```python
from build123d import *

# Parameters (mm, degrees)
F0_W     = 775
F0_H     = 100
F1_DEPTH = 60
F2_W     = 775
F2_H     = 10
F3_DEPTH = 65


with BuildPart() as f1:
    # F0 (on Front) → F1 (new body)
    with BuildSketch(Plane.XZ):
        Polygon((-231.40455, 951.369763), (-301.40455, 951.369763), (-301.40455, -998.630237), (-231.40455, -998.630237), (-231.40455, -898.630237), (-231.40455, -73.630237), (-231.40455, 26.369763), (-231.40455, 851.369763), align=None)
        with Locations((156.09545, 901.369763)):
            Rectangle(F0_W, F0_H)
        Polygon((613.59545, 951.369763), (543.59545, 951.369763), (543.59545, 851.369763), (543.59545, 26.369763), (543.59545, -73.630237), (543.59545, -898.630237), (543.59545, -998.630237), (613.59545, -998.630237), align=None)
        with Locations((156.09545, -23.630237)):
            Rectangle(F0_W, F0_H)
        with Locations((156.09545, -948.630237)):
            Rectangle(F0_W, F0_H)
    extrude(amount=F1_DEPTH)

    # F2 (on Front) → F3 (join)
    with BuildSketch(Plane.XZ):
        Polygon((-241.40455, 16.369763), (-231.40455, 16.369763), (-231.40455, 26.369763), (-231.40455, 851.369763), (-231.40455, 861.369763), (-241.40455, 861.369763), align=None)
        with Locations((156.09545, 21.369763)):
            Rectangle(F2_W, F2_H)
        Polygon((543.59545, 26.369763), (543.59545, 16.369763), (553.59545, 16.369763), (553.59545, 861.369763), (543.59545, 861.369763), (543.59545, 851.369763), align=None)
        with Locations((156.09545, 856.369763)):
            Rectangle(F2_W, F2_H)
    extrude(amount=F3_DEPTH)


solid = f1.part
```
Geometry check sheet. Reference: the model listing, model coordinates, mm. A direction names the side the tool comes from. Coordinates: 2 decimals unless noted, no trailing zeros. Order: outer loops, then holes, each group sorted by start corner. A loop starts at its lowest first (then second) coordinate and runs counter-clockwise, first axis right, second up.
Item 1: Section check C-C (y = -44.5). Enter the section's corners in (x, z).
Item 2: Depth check by flat-ended pin: pin 1 (2.5 mm diameter, centred on y = -62.5, z = 605.5, fed in from +X); pin 2 (1.5 mm diameter, centred on y = -62, z = 372, fed in from -X). Enter the tip coordinate at first touch or a pass-through.
Item 3: Scan lines: line 1 along Z through (x, y) = (3.5, -57.5); line 2 along X through (y, z) = (-42.5, 430.5); line 3 along Y through (x, z) = (-264, -40.5). Record each from-to range of solid material in increasing order.
Item 4: Section check A-A (z = 545.5). Enter the section's corners in (x, y), plus the area to 3 significant figures.
Item 5: Mould release check, pull along X, two halves, no side actions. Record for faces 3 (the flat face through (163, -30, 951.37)), 4 (the flat face through (151, -32, 26.37)), 5 (the flat face through (613.595, -30, -37)): released by +X, released by -X, zero draft, split by the parting line, or undercut.
Item 6: Tool access check on faces 1 (the flat face through (543.595, -30, -480)), 2 (the flat face through (150, -30, -998.63)). Record the directions out of +Z, -Z, +X, -X, +Y, -Y that give a thin tool (end or side, any length) a straight path to the whole face; none if there is none.
Item 7: Section check D-D (z = -319.5). Enter the section's corners in (x, y), plus the area to 3 significant figures.
Item 8: Section check B-B (x = 176). Enter the section's corners in (y, z).
Check sheet entries:
1. outline: (-301.4, -998.63) - (613.6, -998.63) - (613.6, 951.37) - (-301.4, 951.37) - close; hole (-231.4, -898.63) - (543.6, -898.63) - (543.6, -73.63) - (-231.4, -73.63) - close; hole (-231.4, 26.37) - (543.6, 26.37) - (543.6, 851.37) - (-231.4, 851.37) - close
2. pin 1: stops at x = 553.6
2. pin 2: stops at x = -241.4
3. line 1: z = -998.63 to -898.63, -73.63 to 26.37, 851.37 to 951.37
3. line 2: x = -301.4 to -231.4, 543.6 to 613.6
3. line 3: y = -60 to 0
4. outline: (-301.4, -60) - (-241.4, -60) - (-241.4, -65) - (-231.4, -65) - (-231.4, 0) - (-301.4, 0) - close; (543.6, -65) - (553.6, -65) - (553.6, -60) - (613.6, -60) - (613.6, 0) - (543.6, 0) - close
4. area: 8,500 mm2
5. face 3: zero draft
5. face 4: undercut
5. face 5: released by +X
6. face 1: +Y, -Y
6. face 2: -Z, +X, -X, +Y, -Y
7. outline: (-301.4, -60) - (-231.4, -60) - (-231.4, 0) - (-301.4, 0) - close; (543.6, -60) - (613.6, -60) - (613.6, 0) - (543.6, 0) - close
7. area: 8,400 mm2
8. outline: (-65, 16.37) - (-60, 16.37) - (-60, -73.63) - (0, -73.63) - (0, 26.37) - (-65, 26.37) - close; (-65, 851.37) - (0, 851.37) - (0, 951.37) - (-60, 951.37) - (-60, 861.37) - (-65, 861.37) - close; (-60, -998.63) - (0, -998.63) - (0, -898.63) - (-60, -898.63) - close
